from build123d import *

# Parameters (mm, degrees)
SKETCH_1_W          = 50
SKETCH_1_H          = 30
EXTRUDE_1_DEPTH     = 2
SKETCH_2_R          = 2.75
SKETCH_2_R_2        = 1.75
CUT_EXTRUDE_1_DEPTH = 3


with BuildPart() as part:
    # 草图1 → 凸台-拉伸1 (new body)
    with BuildSketch(Plane(origin=(0, 0, 0), x_dir=(1, 0, 0), z_dir=(0, 1, 0))):
        with Locations((25, 15)):
            Rectangle(SKETCH_1_W, SKETCH_1_H)
    extrude(amount=EXTRUDE_1_DEPTH)

    # 草图2 → 切除-拉伸1 (cut, through all)
    with BuildSketch(Plane(origin=(0, 2, 0), x_dir=(1, 0, 0), z_dir=(0, 1, 0))):
        with Locations((40, 6)):
            Circle(SKETCH_2_R)
        with Locations((12, 15)):
            Circle(SKETCH_2_R_2)
        with Locations((40, 24)):
            Circle(SKETCH_2_R)
        Polygon((0, 7.071067812), (7.071067812, 0), (0, 0), align=None)
    extrude(amount=-CUT_EXTRUDE_1_DEPTH, mode=Mode.SUBTRACT)


solid = part.part
Input: part model. Units: mm. Frame: model coordinates. Round coordinates to 2 decimals unless told otherwise and drop trailing zeros. Write each loop counter-clockwise with the first axis right and the second up, starting at its lowest first coordinate (ties: lowest second). Pieces come first, ordered by that corner, then holes.
1) Draft query along Z for faces 1 (the cylindrical face through (37.253, 1.014, -24.121)), 2 (the flat face through (25, 0, -15)), 3 (the cylindrical face through (37.253, 1.014, -6.121)), 4 (the flat face through (28, 1, 0)). Return one class per face: pulls with the +Z half, pulls with the -Z half, needs draft (parallel to the pull), parting line crosses it, or undercut.
2) Ray query, L1, parallel to Z at x = 40, y = 0.9; L2, parallel to X at y = 1.25, z = -24; L3, parallel to X at y = 1.4, z = -15. Return the intervals inside material, ascending.
3) Cut plane C-C (y = 1.05). Return the cut outline in (x, z).
4) Cut plane A-A (z = -24). Return the cut outline in (x, y), then the cut area to 3 significant figures.
5) Cut plane B-B (x = 40). Return the cut outline in (y, z).
6) Cut plane D-D (z = -15). Return the cut outline in (x, y), then the cut area to 3 significant figures.
Geometry says:
1. face 1: undercut
1. face 2: needs draft
1. face 3: undercut
1. face 4: pulls with the +Z half
2. L1: z = -30 to -26.75, -21.25 to -8.75, -3.25 to 0
2. L2: x = 0 to 37.25, 42.75 to 50
2. L3: x = 0 to 10.25, 13.75 to 50
3. outline: (0, -30) - (50, -30) - (50, 0) - (7.07, 0) - (0, -7.07) - close; hole circle Ø3.5 at (12, -15); hole circle Ø5.5 at (40, -24); hole circle Ø5.5 at (40, -6)
4. outline: (0, 0) - (37.25, 0) - (37.25, 2) - (0, 2) - close; (42.75, 0) - (50, 0) - (50, 2) - (42.75, 2) - close
4. area: 89.0 mm2
5. outline: (0, -30) - (2, -30) - (2, -26.75) - (0, -26.75) - close; (0, -21.25) - (2, -21.25) - (2, -8.75) - (0, -8.75) - close; (0, -3.25) - (2, -3.25) - (2, 0) - (0, 0) - close
6. outline: (0, 0) - (10.25, 0) - (10.25, 2) - (0, 2) - close; (13.75, 0) - (50, 0) - (50, 2) - (13.75, 2) - close
6. area: 93.0 mm2
